Geometry check sheet. Reference: the model listing, model coordinates, mm. Face numbers are marked on the shaded views. A direction names the side the tool comes from. Give positions to 0.01 mm unless a question says otherwise; leave off trailing zeros. Write each loop counter-clockwise with the first axis right and the second up, starting at its lowest first coordinate (ties: lowest second). Pieces come first, ordered by that corner, then holes. Notation, with made-up numbers: M 31.25,38.25 L 69.25,38.25 A16 cw 69.25,68.25 Z; hole C -0.5,51.25 d1. An arc over 180 degrees is marked long. One line per item, written item: value. Start each with the question number.
1. Cross-section at A-A on y = 0. Record the cut outline in (x, z), then the cut area to 3 significant figures.
2. Release check for a two-part mould opening along Y. For the marked faces 3, 4, 5 and 6 record: pulls with the +Y half, pulls with the -Y half, needs draft (parallel to the pull), parting line crosses it, or undercut.
3. Cross-section at B-B on x = 0. Record the cut outline in (y, z), then the cut area to 3 significant figures.
4. Gauge pin test, flat end, axial feed: pin 1 (1 mm diameter, centred on x = -2, z = 3.5, fed in from -Y). Record the tip position at first contact, or that the pin passes through.
5. Tool access check on the marked faces 1 and 2. Record the directions out of +Z, -Z, +X, -X, +Y, -Y that give a thin tool (end or side, any length) a straight path to the whole face; none if there is none.
6. Cross-section at D-D on z = 0.4. Record the cut outline in (x, y) (3 decimals), then the cut area to 3 significant figures.
7. Scan lines: line 1 (X direction, y = 0, z = 3.75); line 2 (Z direction, x = 0.75, y = -2.5); line 3 (Y direction, x = -1, z = 1.85). Record each from-to range of solid material in increasing order.
8. Cross-section at C-C on z = 3.8. Record the cut outline in (x, y) (3 decimals), then the cut area to 3 significant figures.
from build123d import *

# Parameters (mm, degrees)
F1_DEPTH = 5
F3_DEPTH = 1
F4_SIZE  = 0.4


with BuildPart() as f1:
    # F0 (on Top) → F1 (new body)
    with BuildSketch(Plane.XY):
        with BuildLine():
            ThreePointArc((-1.726239, 4.01), (-2.144514, 3.402767), (-2.647546, 2.863652))
            ThreePointArc((-2.647546, 2.863652), (0, -3.9), (2.647546, 2.863652))
            ThreePointArc((2.647546, 2.863652), (2.144514, 3.402767), (1.726239, 4.01))
            ThreePointArc((1.726239, 4.01), (0, 5), (-1.726239, 4.01))
        make_face()
        with BuildLine():
            ThreePointArc((1.999097, 2.236875), (0, -3), (-1.999097, 2.236875))
            ThreePointArc((-1.999097, 2.236875), (-1.425915, 2.842359), (-0.961315, 3.534672))
            ThreePointArc((-0.961315, 3.534672), (0, 4.1), (0.961315, 3.534672))
            ThreePointArc((0.961315, 3.534672), (1.425915, 2.842359), (1.999097, 2.236875))
        make_face(mode=Mode.SUBTRACT)
    extrude(amount=F1_DEPTH)

    # F2 (on Top) → F3 (join)
    with BuildSketch(Plane.XY):
        with BuildLine():
            ThreePointArc((-0.961315, 3.534672), (-1.425915, 2.842359), (-1.999097, 2.236875))
            ThreePointArc((-1.999097, 2.236875), (0, -3), (1.999097, 2.236875))
            ThreePointArc((1.999097, 2.236875), (1.425915, 2.842359), (0.961315, 3.534672))
            ThreePointArc((0.961315, 3.534672), (0, 4.1), (-0.961315, 3.534672))
        make_face()
    extrude(amount=F3_DEPTH)

    # F4
    f4_edges = [f1.edges().sort_by_distance(p)[0] for p in [
        (0, -3, 5),
    ]]
    chamfer(f4_edges, length=F4_SIZE)


solid = f1.part
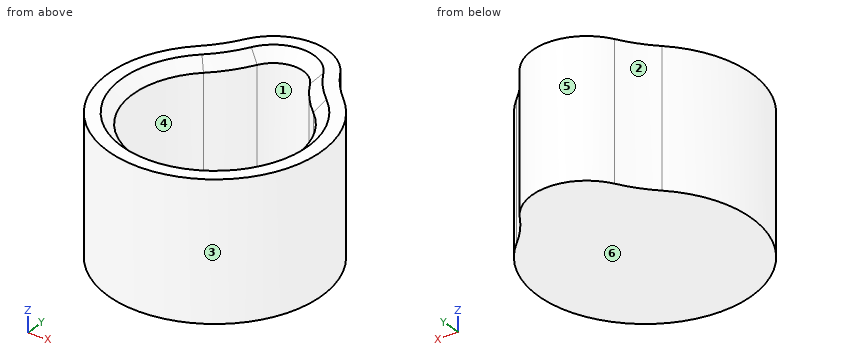
Report:
1. outline: M -3.9,0 L 3.9,0 L 3.9,5 L 3.4,5 L 3,4.6 L 3,1 L -3,1 L -3,4.6 L -3.4,5 L -3.9,5 Z
1. area: 14.8 mm^2
2. face 3: parting line crosses it
2. face 4: undercut
2. face 5: pulls with the +Y half
2. face 6: needs draft
3. outline: M -3.9,0 L 5,0 L 5,5 L 4.5,5 L 4.1,4.6 L 4.1,1 L -3,1 L -3,4.6 L -3.4,5 L -3.9,5 Z
3. area: 15.9 mm^2
4. pin 1: stops at y = -3.6
5. face 1: +Z
5. face 2: +Z, -Z, -X, +Y
6. outline: M -2.648,2.864 A3.9 ccw long 2.648,2.864 A5 cw 1.726,4.01 A2 ccw -1.726,4.01 A5 cw Z
6. area: 51.3 mm^2
7. line 1: x = -3.9 to -3, 3 to 3.9
7. line 2: z = 0 to 1
7. line 3: y = -3.77 to -2.83, 3.47 to 4.73
8. outline: M -2.648,2.864 A3.9 ccw long 2.648,2.864 A5 cw 1.726,4.01 A2 ccw -1.726,4.01 A5 cw Z; hole M -1.999,2.237 A3 ccw long 1.999,2.237 A5 cw 0.961,3.535 A1.1 ccw -0.961,3.535 A5 cw Z
8. area: 20.7 mm^2
